```python
from build123d import *

# Parameters (mm, degrees)
ESQUISSE1_W        = 19.15
ESQUISSE1_H        = 55.52
BOSS_EXTRU_1_DEPTH = 25
ESQUISSE3_R        = 1.46
BOSS_EXTRU_2_DEPTH = 46.45


with BuildPart() as part:
    # Esquisse1 → Boss.-Extru.1 (new body)
    with BuildSketch(Plane(origin=(0, 0, 0), x_dir=(1, 0, 0), z_dir=(0, 1, 0))):
        with Locations((9.575, 27.76)):
            Rectangle(ESQUISSE1_W, ESQUISSE1_H)
    extrude(amount=BOSS_EXTRU_1_DEPTH)

    # Esquisse3 → Boss.-Extru.2 (add)
    with BuildSketch(Plane(origin=(0, 0, 0), x_dir=(0, 0, -1), z_dir=(1, 0, 0))):
        with Locations((49.726650103, 12.5)):
            Circle(ESQUISSE3_R)
    extrude(amount=BOSS_EXTRU_2_DEPTH)


solid = part.part
```
Build history of the part. All positions in model axes, mm. A direction names the side the tool comes from. Coordinates: 2 decimals unless noted, no trailing zeros. Order: outer loops, then holes, each group sorted by start corner. A loop starts at its lowest first (then second) coordinate and runs counter-clockwise, first axis right, second up.
Item 1: Drop flat-ended pins along their axis: pin 1 Ø6 at (x, y) = (32, 12) entering from -Z; pin 2 Ø12.5 at (y, z) = (15.5, -20) entering from +X; pin 3 Ø10 at (x, z) = (36.5, -50) entering from -Y. Give the stop position or say it passes through.
Filled in:
pin 1: stops at z = -51.19
pin 2: stops at x = 19.15
pin 3: stops at y = 11.04
Item 2: Saw through at D-D on y = 5. List the corners of the cut face in (x, z), then the cut area to 3 significant figures.
Filled in:
outline: (0, -55.52) - (19.15, -55.52) - (19.15, 0) - (0, 0) - close
area: 1,060 mm2
Item 3: Drill centre line: L1, parallel to X at y = 12.5, z = -21. Where is it in solid material? Low to high.
Filled in:
L1: x = 0 to 19.15
Item 4: Saw through at B-B on z = -30. List the corners of the cut face in (x, y), then the cut area to 3 significant figures.
Filled in:
outline: (0, 0) - (19.15, 0) - (19.15, 25) - (0, 25) - close
area: 479 mm2
Item 5: Tool access for faces 1 (the flat face through (9, 25, -28)), 2 (the cylindrical face through (32.609, 11.205, -50.4)): list every direction of +Z, -Z, +X, -X, +Y, -Y with a clear straight run to the whole face (end or side of a thin tool).
Filled in:
face 1: +Z, -Z, +X, -X, +Y
face 2: +X
Item 6: Saw through at A-A on y = 12.5. List the corners of the cut face in (x, z).
Filled in:
outline: (0, -55.52) - (19.15, -55.52) - (19.15, -51.19) - (46.45, -51.19) - (46.45, -48.27) - (19.15, -48.27) - (19.15, 0) - (0, 0) - close
Item 7: Saw through at C-C on x = 34. List the corners of the cut face in (y, z).
Filled in:
outline: circle Ø2.92 at (12.5, -49.73)
